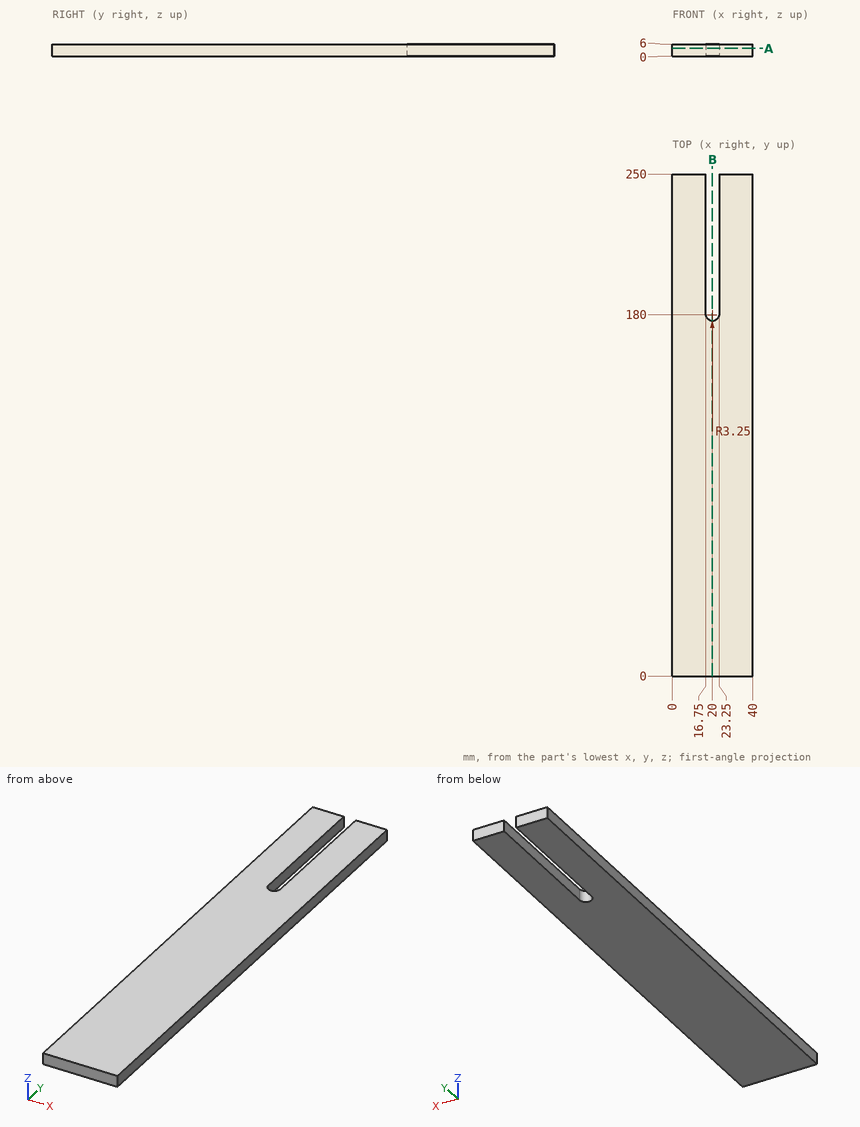
Answer from the drawing. Dimensions are ordinates in mm from the lowest x, y and z of the part. Give positions to 0.01 mm unless a question says otherwise; leave off trailing zeros. Write each loop counter-clockwise with the first axis right and the second up, starting at its lowest first coordinate (ties: lowest second). Pieces come first, ordered by that corner, then holes. Notation, with made-up numbers: (89, -13) - (125, -13) arc R16 cw to (125, 8) - close; hole circle Ø3 at (21, -12). An arc over 180 degrees is marked (long way). One line per item, written item: value. Start each with the question number.
1. Find section B-B (x = 20). Write down the section's boundary in (y, z), then the cut area to 3 significant figures.
2. Given pin 1 (1 mm diameter, centred on x = 18.5, z = 3.5, fed in from +Y), flat-ended and moving along its own axis, determine where the tip first touches the part or whether it passes through.
3. Find section A-A (z = 3.85). Write down the section's boundary in (x, y), then the cut area to 3 significant figures.
4. Consider probe 1 along X at (y, z) = (199, 0.7); probe 2 along Y at (x, z) = (17.5, 5.7). Determine where each line is inside the solid, lowest interval first.
Geometry results:
1. outline: (0, 0) - (176.75, 0) - (176.75, 6) - (0, 6) - close
1. area: 1,060 mm2
2. pin 1: y = 177.44
3. outline: (0, 0) - (40, 0) - (40, 250) - (23.25, 250) - (23.25, 180) arc R3.25 cw to (16.75, 180) - (16.75, 250) - (0, 250) - close
3. area: 9,530 mm2
4. probe 1: 0 to 16.75, 23.25 to 40
4. probe 2: 0 to 177.92
